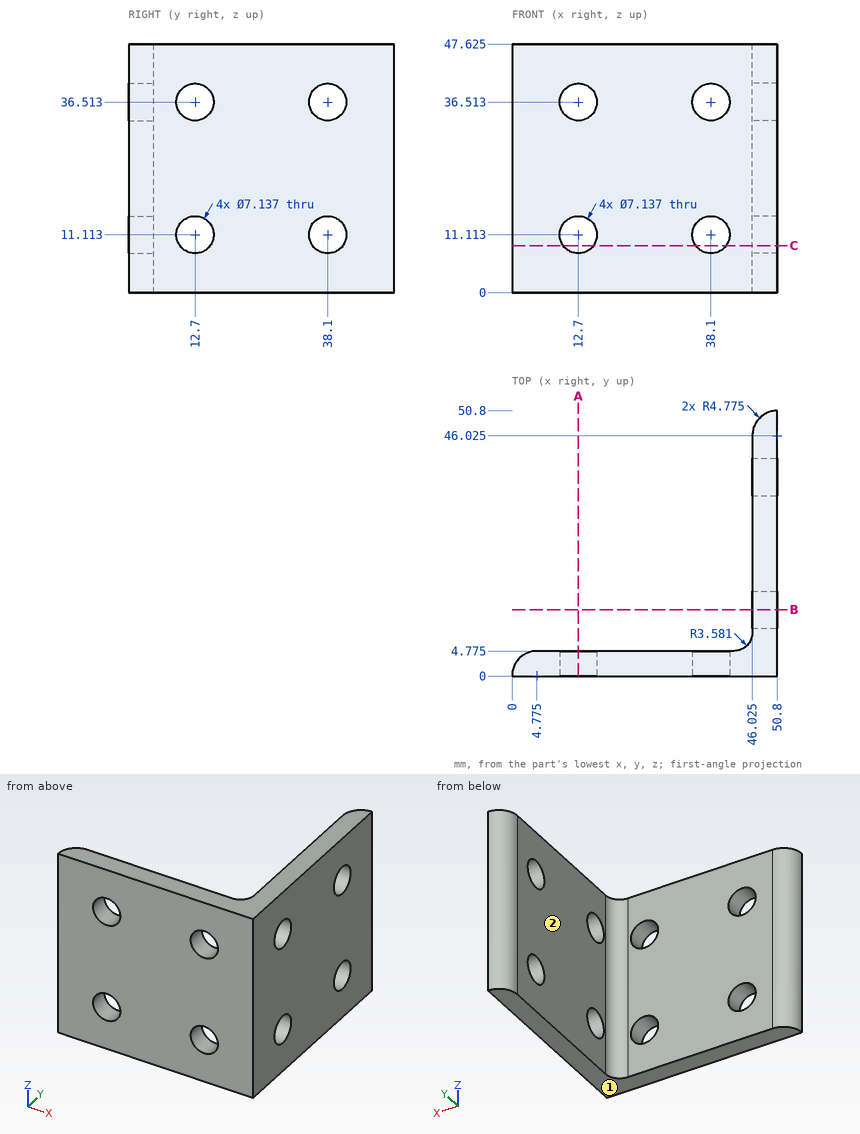
Geometry: see drawing. Coordinates: mm, zero at the bounding-box minimum. A direction names the side the tool comes from. Round coordinates to 2 decimals unless told otherwise and drop trailing zeros. Write each loop counter-clockwise with the first axis right and the second up, starting at its lowest first coordinate (ties: lowest second). Pieces come first, ordered by that corner, then holes.
Item 1: Section query B-B (y = 12.7). Return loops of the section in (x, z) (1 decimal), plus the area to 3 significant figures.
Item 2: Set-up query: the marked faces 1 and 2. Return all of +Z, -Z, +X, -X, +Y, -Y with unobstructed straight access to the full face (end or side cutting, diameter ignored); none if empty.
Item 3: Material intervals for L1, parallel to Z at x = 49.1, y = 12.7 (1 decimal); L2, parallel to Z at x = 10, y = 4 (1 decimal); L3, parallel to X at y = 15.5, z = 27.5 (1 decimal), sorted ascending.
Item 4: Pin query (flat end, axial travel): P1, Ø11.5, axis at y = 26.5, z = 20, coming from the -X side (1 decimal); P2, Ø1.5, axis at x = 28, z = 15, coming from the +Y side (1 decimal). Return the tip coordinate at first contact, or that it passes through.
Item 5: Section query C-C (z = 9). Give the number of separate pieces and of enclosed holes in the cut face.
Item 6: Section query A-A (x = 12.7). Return loops of the section in (y, z) (1 decimal), plus the area to 3 significant figures.
Completed:
1. outline: (46, 0) - (50.8, 0) - (50.8, 7.5) - (46, 7.5) - close; (46, 14.7) - (50.8, 14.7) - (50.8, 32.9) - (46, 32.9) - close; (46, 40.1) - (50.8, 40.1) - (50.8, 47.6) - (46, 47.6) - close
1. area: 159 mm2
2. face 1: -Z, +X, -X, +Y, -Y
2. face 2: +Z, -Z, -X, +Y
3. L1: z = 0 to 7.5, 14.7 to 32.9, 40.1 to 47.6
3. L2: z = 0 to 8.8, 13.4 to 34.2, 38.8 to 47.6
3. L3: x = 46 to 50.8
4. P1: stops at x = 46
4. P2: stops at y = 4.8
5. separate pieces: 5
5. enclosed holes: 0
6. outline: (0, 0) - (4.8, 0) - (4.8, 7.5) - (0, 7.5) - close; (0, 14.7) - (4.8, 14.7) - (4.8, 32.9) - (0, 32.9) - close; (0, 40.1) - (4.8, 40.1) - (4.8, 47.6) - (0, 47.6) - close
6. area: 159 mm2
